```python
from build123d import *

# Parameters (mm, degrees)
SKETCH_1_R          = 21
EXTRUDE_1_DEPTH     = 17
SKETCH_2_R          = 8
EXTRUDE_2_DEPTH     = 1.5
SKETCH_3_R          = 3
EXTRUDE_3_DEPTH     = 20.5
CHAMFER_1_SIZE      = 1
THREAD_1_PITCH      = 1
CUT_EXTRUDE_1_DEPTH = 1
EXTRUDE1_DEPTH      = 50.020403995
EXTRUDE1_DEPTH_BACK = 50.020403995
SKETCH1_W           = 6
SKETCH1_H           = 20.5
SKETCH2_R           = 2
EXTRUDE2_DEPTH      = 20
FILLET1_R           = 0.5
SKETCH3_R           = 1
EXTRUDE3_DEPTH      = 2
FILLET2_R           = 0.5
EXTRUDE5_START      = -0.5
SKETCH4_R           = 5
SKETCH4_R_2         = 2
EXTRUDE5_DEPTH      = 0.5
SKETCH5_R           = 21.25
EXTRUDE7_DEPTH      = 17
SKETCH6_W           = 16
SKETCH6_H           = 3
EXTRUDE8_DEPTH      = 8
SKETCH7_W           = 15
SKETCH7_H           = 2
EXTRUDE9_DEPTH      = 3


with BuildPart() as part:
    # Sketch 1 → 보스-돌출1 (new body)
    with BuildSketch(Plane.XY):
        Circle(SKETCH_1_R)
    extrude(amount=EXTRUDE_1_DEPTH)

    # 스케치2 → 보스-돌출2 (add)
    with BuildSketch(Plane.XY.offset(17)):
        Circle(SKETCH_2_R)
    extrude(amount=EXTRUDE_2_DEPTH)

    # 스케치3 → 보스-돌출3 (add)
    with BuildSketch(Plane.XY.offset(18.5)):
        Circle(SKETCH_3_R)
    extrude(amount=EXTRUDE_3_DEPTH)

    # 모따기1
    chamfer_1_edges = [part.edges().sort_by_distance(p)[0] for p in [
        (-3, 0, 39),
    ]]
    chamfer(chamfer_1_edges, length=CHAMFER_1_SIZE)

    # 나사산1: the profile of Sketch 1 2 profile screwed along a right-hand helix of 8 turns, 8 arcs to a turn; built about Z, then put on its axis
    thread_1_z = Axis((0, 0, 0), (0, 0, 1))
    thread_1_corners = [(3.0003, 0, -0.000173205), (3.0003, 0, 0.875173202), (2.458734125, 0, 0.562499999), (2.458734125, 0, 0.312499999)]
    with BuildLine(mode=Mode.PRIVATE) as thread_1_profile:
        Line(thread_1_corners[0], thread_1_corners[1])
        Line(thread_1_corners[1], thread_1_corners[2])
        Line(thread_1_corners[2], thread_1_corners[3])
        Line(thread_1_corners[3], thread_1_corners[0])
    thread_1_cap = Face(thread_1_profile.wire())
    thread_1_turn_angles = [0, 22.5, 45, 67.5, 90, 112.5, 135, 157.5, 180, 202.5, 225, 247.5, 270, 292.5, 315, 337.5, 360]
    thread_1_turn_weights = [1, 0.9238795325112867, 1, 0.9238795325112867, 1, 0.9238795325112867, 1, 0.9238795325112867, 1, 0.9238795325112867, 1, 0.9238795325112867, 1, 0.9238795325112867, 1, 0.9238795325112867, 1]
    thread_1_turn_rails = [Edge.make_bspline([Vector(p[0], p[1], 0).rotate(thread_1_z, thread_1_turn_angles[k]) / thread_1_turn_weights[k] + Vector(0, 0, p[2] + THREAD_1_PITCH * thread_1_turn_angles[k] / 360) for k in range(17)], [0, 0, 0, 1, 1, 2, 2, 3, 3, 4, 4, 5, 5, 6, 6, 7, 7, 8, 8, 8], 2, thread_1_turn_weights) for p in thread_1_corners]
    thread_1_turn_sides = [Face.make_surface_from_curves(thread_1_turn_rails[p[0]], thread_1_turn_rails[p[1]]) for p in [(0, 1), (1, 2), (2, 3), (3, 0)]]
    thread_1 = Plane(origin=(0, 0, 38), x_dir=(-1, 0, 0), z_dir=(0, 0, -1)) * Solid(Shell([*[p.moved(Location((0, 0, THREAD_1_PITCH * i))) for i in range(8) for p in thread_1_turn_sides], thread_1_cap, thread_1_cap.rotate(thread_1_z, 2880).moved(Location((0, 0, THREAD_1_PITCH * 2880 / 360)))]))
    add(thread_1, mode=Mode.SUBTRACT)

    # 스케치8 → 컷-돌출1 (cut)
    with BuildSketch(Plane(origin=(0, 3, 0), x_dir=(1, 0, 0), z_dir=(0, 1, 0))):
        Polygon((3, -39), (3, -38), (3, -37.5), (3, -29.625000003), (3, -27), (-3, -27), (-3, -29.125000003), (-3, -30), (-3, -37.125000003), (-3, -38), (-3, -39), (-2, -39), (2, -39), align=None)
    extrude(amount=-CUT_EXTRUDE_1_DEPTH, mode=Mode.SUBTRACT)

    # Sketch1 → Extrude1 (cut, two sides: drawn at the far end of the back side and taken through both)
    with BuildSketch(Plane(origin=(0, 0, 0), x_dir=(1, 0, 0), z_dir=(0, 1, 0)).offset(-EXTRUDE1_DEPTH_BACK)):
        with Locations((0, -28.75)):
            Rectangle(SKETCH1_W, SKETCH1_H)
    extrude(amount=EXTRUDE1_DEPTH + EXTRUDE1_DEPTH_BACK, mode=Mode.SUBTRACT)

    # Sketch2 → Extrude2 (add)
    with BuildSketch(Plane.XY.offset(18.5)):
        Circle(SKETCH2_R)
    extrude(amount=EXTRUDE2_DEPTH)

    # Fillet1
    fillet1_edges = [part.edges().sort_by_distance(p)[0] for p in [
        (-2, 0, 38.5),
    ]]
    fillet(fillet1_edges, radius=FILLET1_R)

    # Sketch3 → Extrude3 (cut)
    with BuildSketch(Plane.XY.offset(38.5)):
        Circle(SKETCH3_R)
    extrude(amount=-EXTRUDE3_DEPTH, mode=Mode.SUBTRACT)

    # Fillet2
    fillet2_edges = [part.edges().sort_by_distance(p)[0] for p in [
        (-1, 0, 36.5),
    ]]
    fillet(fillet2_edges, radius=FILLET2_R)

    # Sketch4 → Extrude5 (cut)
    with BuildSketch(Plane.XY.offset(18.5).offset(EXTRUDE5_START)):
        Circle(SKETCH4_R)
        Circle(SKETCH4_R_2, mode=Mode.SUBTRACT)
    extrude(amount=EXTRUDE5_DEPTH, mode=Mode.SUBTRACT)

    # Sketch5 → Extrude7 (add)
    with BuildSketch(Plane(origin=(0, 0, 0), x_dir=(-1, 0, 0), z_dir=(0, 0, -1))):
        Circle(SKETCH5_R)
    extrude(amount=EXTRUDE7_DEPTH)

    # Sketch6 → Extrude8 (add)
    with BuildSketch(Plane(origin=(0, 15, 0), x_dir=(1, 0, 0), z_dir=(0, 1, 0))):
        with Locations((0, 6.5)):
            Rectangle(SKETCH6_W, SKETCH6_H)
    extrude(amount=EXTRUDE8_DEPTH)

    # Sketch7 → Extrude9 (cut)
    with BuildSketch(Plane(origin=(0, 23, 0), x_dir=(1, 0, 0), z_dir=(0, 1, 0))):
        with Locations((0, 6.5)):
            Rectangle(SKETCH7_W, SKETCH7_H)
    extrude(amount=-EXTRUDE9_DEPTH, mode=Mode.SUBTRACT)


solid = part.part
```
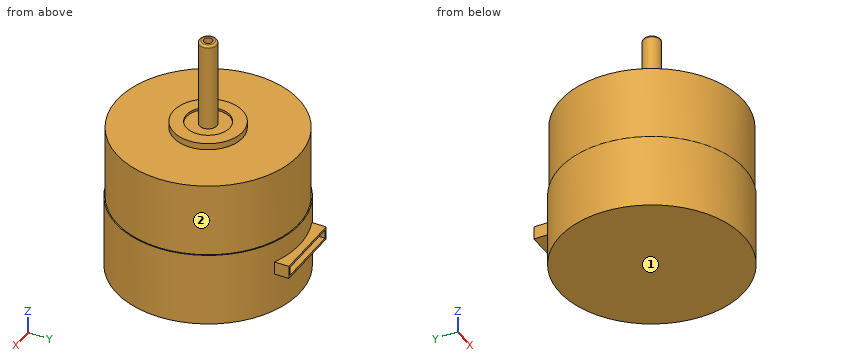
Geometry: final body of the model. Coordinates: model frame, mm. Face numbers are marked on the shaded views. A direction names the side the tool comes from. Round coordinates to 2 decimals unless told otherwise and drop trailing zeros. Write each loop counter-clockwise with the first axis right and the second up, starting at its lowest first coordinate (ties: lowest second). Pieces come first, ordered by that corner, then holes. Notation, with made-up numbers: (40, 38) -> (78, 38) arc R32 ccw to (78, 72) -> close; hole circle Ø3 at (86.25, 82.5). An arc over 180 degrees is marked (long way). Use CSV: the item, a comma, the result in double quotes. Start each with the question number.
Q1. Section A-A (y = 17). Return loops of the section in (x, z).
Q2. Section D-D (y = -3.5). Return loops of the section in (x, z), plus the area to 3 significant figures.
Q3. Section C-C (z = -12). Return loops of the section in (x, y), plus the area to 3 significant figures.
Q4. Line query: L1, parallel to Y at x = 0, z = 18.4; L2, parallel to Y at x = 0, z = 37; L3, parallel to Z at x = 2.5, y = -7. Output: solid intervals per line, ascending.
Q5. Section B-B (x = -15.5). Return loops of the section in (y, z).
Q6. First-contact query: pin 1 Ø2.5 at (y, z) = (20.5, -6) entering from -X; pin 2 Ø0.5 at (x, y) = (0, 0) entering from +Z; pin 3 Ø3 at (y, z) = (-6, 14) entering from +X; pin 4 Ø1 at (x, z) = (-13, 19) entering from -Y. Flat tips, straight axial feed; report the tip coordinate or a pass-through.
Q7. Reachability of the marked faces 1 and 2 from +Z, -Z, +X, -X, +Y, -Y: full face, straight path, thin tool, end or side. Return the list, or none.
Result sheet:
1,outline,"(-12.75, -17) -> (12.75, -17) -> (12.75, 0) -> (12.33, 0) -> (12.33, 17) -> (-12.33, 17) -> (-12.33, 0) -> (-12.75, 0) -> close"
2,outline,"(-20.96, -17) -> (20.96, -17) -> (20.96, 0) -> (20.71, 0) -> (20.71, 17) -> (7.19, 17) -> (7.19, 18.5) -> (3.57, 18.5) -> (3.57, 18) -> (-3.57, 18) -> (-3.57, 18.5) -> (-7.19, 18.5) -> (-7.19, 17) -> (-20.71, 17) -> (-20.71, 0) -> (-20.96, 0) -> close"
2,area,"1,430 mm²"
3,outline,"circle Ø42.5 at (0, 0)"
3,area,"1,420 mm²"
4,L1,"-8 to -5, -2 to 2, 5 to 8"
4,L2,"-2 to -1, 1 to 2"
4,L3,"-17 to 18.5"
5,outline,"(-14.54, -17) -> (14.54, -17) -> (14.54, 0) -> (14.17, 0) -> (14.17, 17) -> (-14.17, 17) -> (-14.17, 0) -> (-14.54, 0) -> close"
6,pin 1,"x = -9"
6,pin 2,"z = 36.5"
6,pin 3,"x = 20.51"
6,pin 4,"through"
7,face 1,"-Z, +X, -X, +Y, -Y"
7,face 2,"+Z"
